```python
from build123d import *
from build123d.topology import SkipClean

# Parameters (mm, degrees)
SKETCH1_W           = 10
SKETCH1_H           = 10
BOSS_EXTRUDE1_DEPTH = 100
SKETCH2_W           = 25
SKETCH2_H           = 20
SKETCH2_R           = 1
BOSS_EXTRUDE2_DEPTH = 2
CUT_EXTRUDE2_DEPTH  = 2.5
CHAMFER2_SIZE       = 2.5
BOSS_EXTRUDE3_DEPTH = 7.5
CUT_EXTRUDE3_DEPTH  = 7.5
SKETCH8_W           = 40
SKETCH8_H           = 10
BOSS_EXTRUDE4_DEPTH = 3
FILLET1_R           = 2
SKETCH9_R           = 3
CUT_EXTRUDE4_DEPTH  = 5


with BuildPart() as part:
    # Sketch1 → Boss-Extrude1 (new, symmetric)
    with BuildSketch(Plane.XY):
        Rectangle(SKETCH1_W, SKETCH1_H)
    extrude(amount=BOSS_EXTRUDE1_DEPTH, both=True)

    # Sketch2 → Boss-Extrude2 (add)
    with BuildSketch(Plane(origin=(0, 0, -100), x_dir=(-1, 0, 0), z_dir=(0, 0, -1))):
        with Locations((0, 5)):
            Rectangle(SKETCH2_W, SKETCH2_H)
        with Locations((-8, 5.6)):
            Circle(SKETCH2_R, mode=Mode.SUBTRACT)
        with Locations(Location((8, 5.6, 0), (0, 0, 180))):
            Circle(SKETCH2_R, mode=Mode.SUBTRACT)
    extrude(amount=BOSS_EXTRUDE2_DEPTH)

    # Sketch4 → Cut-Extrude2 (cut)
    with BuildSketch(Plane(origin=(0, 5, 0), x_dir=(1, 0, 0), z_dir=(0, 1, 0))):
        Polygon((5, 100), (2.5, 100), (2.5, 92.5), (5, 90), (5, 92.5), align=None)
        Polygon((-5, 90), (-5, 92.5), (-5, 100), (-2.5, 100), (-2.5, 92.5), align=None)
    extrude(amount=-CUT_EXTRUDE2_DEPTH, mode=Mode.SUBTRACT)

    # Chamfer2
    chamfer2_edges = [part.edges().sort_by_distance(p)[0] for p in [
        (-2.5, 2.5, -96.25),
        (2.5, 2.5, -96.25),
    ]]
    chamfer(chamfer2_edges, length=CHAMFER2_SIZE - 0.0001)  # a hair under: the kernel refuses the full size

    # Sketch5 → Boss-Extrude3 (add)
    with SkipClean():  # the faces are left unmerged after this step: merging them gives an invalid solid
        with BuildSketch(Plane.XY.offset(-100)):
            Polygon((-2.5, 5), (-1, 6.5), (1, 6.5), (2.5, 5), align=None)
        extrude(amount=BOSS_EXTRUDE3_DEPTH)

    # Sketch7 → Cut-Extrude3 (cut)
    with SkipClean():  # the faces are left unmerged after this step: merging them gives an invalid solid
        with BuildSketch(Plane(origin=(5, 0, 0), x_dir=(0, 0, -1), z_dir=(1, 0, 0))):
            Polygon((92.5, 5), (94, 6.5), (92.5, 6.5), align=None)
        extrude(amount=-CUT_EXTRUDE3_DEPTH, mode=Mode.SUBTRACT)

    # Chamfer3: read off the stored shape, not the designer's step
    # Chamfer3: loft between two sections, ruled curve by curve
    with SkipClean():  # the faces are left unmerged after this step: merging them gives an invalid solid
        chamfer3_from = [
            Edge.make_line((-5, -5, -98.267949192), (-5, 2.5, -98.267949192)),
            Edge.make_line((-5, 2.5, -98.267949192), (-1, 6.5, -98.267949192)),
            Edge.make_line((-1, 6.5, -98.267949192), (1, 6.5, -98.267949192)),
            Edge.make_line((1, 6.5, -98.267949192), (5, 2.5, -98.267949192)),
            Edge.make_line((5, -5, -98.267949192), (5, 2.5, -98.267949192)),
            Edge.make_line((5, -5, -98.267949192), (-5, -5, -98.267949192)),
        ]
        chamfer3_to = [
            Edge.make_line((-6, -5, -100), (-6, 2.914213562, -100)),
            Edge.make_line((-6, 2.914213562, -100), (-1.414213562, 7.5, -100)),
            Edge.make_line((-1.414213562, 7.5, -100), (1.414213562, 7.5, -100)),
            Edge.make_line((1.414213562, 7.5, -100), (6, 2.914213562, -100)),
            Edge.make_line((6, -5, -100), (6, 2.914213562, -100)),
            Edge.make_line((6, -5, -100), (-6, -5, -100)),
        ]
        chamfer3 = Solid(Shell([*[Face.make_surface_from_curves(chamfer3_from[k], chamfer3_to[k]) for k in range(6)], Face(Wire(chamfer3_from)), Face(Wire(chamfer3_to))]))
        add(chamfer3)

    # Sketch8 → Boss-Extrude4 (add)
    with SkipClean():  # the faces are left unmerged after this step: merging them gives an invalid solid
        with BuildSketch(Plane(origin=(5, 0, 0), x_dir=(0, 0, -1), z_dir=(1, 0, 0))):
            Rectangle(SKETCH8_W, SKETCH8_H)
            with BuildLine():
                Line((0.419781931, 3.827046267), (16.278971963, 2.087479782))
                ThreePointArc((16.278971963, 2.087479782), (18.15, 0), (16.278971963, -2.087479782))
                Line((16.278971963, -2.087479782), (0.419781931, -3.827046267))
                ThreePointArc((0.419781931, -3.827046267), (0, -3.85), (-0.419781931, -3.827046267))
                Line((-0.419781931, -3.827046267), (-16.278971963, -2.087479782))
                ThreePointArc((-16.278971963, -2.087479782), (-18.15, 0), (-16.278971963, 2.087479782))
                Line((-16.278971963, 2.087479782), (-0.419781931, 3.827046267))
                ThreePointArc((-0.419781931, 3.827046267), (0, 3.85), (0.419781931, 3.827046267))
            make_face(mode=Mode.SUBTRACT)
        extrude(amount=BOSS_EXTRUDE4_DEPTH)

    # Fillet1
    # the kernel refuses this fillet: 2 mm, written as the material it takes off along each edge
    with BuildSketch(Plane(origin=(5, 5, -20), x_dir=(0, -1, 0), z_dir=(1, 0, 0)), Plane(origin=(5, -5, -20), x_dir=(0, 0, 1), z_dir=(1, 0, 0))) as fillet1_piece_1:
        with BuildLine():
            CenterArc((FILLET1_R, -FILLET1_R), FILLET1_R, 90, 90)
            Line((0, -FILLET1_R), (0, 0))
            Line((0, 0), (FILLET1_R, 0))
        make_face()
    extrude(amount=8, mode=Mode.SUBTRACT)
    with BuildSketch(Plane(origin=(5, 5, 20), x_dir=(0, -1, 0), z_dir=(1, 0, 0)), Plane(origin=(5, -5, 20), x_dir=(0, 0, -1), z_dir=(1, 0, 0))) as fillet1_piece_2:
        with BuildLine():
            CenterArc((FILLET1_R, FILLET1_R), FILLET1_R, 180, 90)
            Line((0, FILLET1_R), (0, 0))
            Line((0, 0), (FILLET1_R, 0))
        make_face()
    extrude(amount=8, mode=Mode.SUBTRACT)

    # Sketch9 → Cut-Extrude4 (cut)
    with SkipClean():  # the faces are left unmerged after this step: merging them gives an invalid solid
        with BuildSketch(Plane.ZY.offset(5)):
            Circle(SKETCH9_R)
        extrude(amount=-CUT_EXTRUDE4_DEPTH, mode=Mode.SUBTRACT)


solid = part.part
```
For this review, take the finished solid that the model builds, in its own axes (mm). A direction names the side the tool comes from. Round coordinates to 2 decimals unless told otherwise and drop trailing zeros. Write each loop counter-clockwise with the first axis right and the second up, starting at its lowest first coordinate (ties: lowest second). Pieces come first, ordered by that corner, then holes. Notation, with made-up numbers: (-24.5, 78.5) - (-16.5, 78.5) arc R14 cw to (-16.5, 89.5) - close; hole circle Ø4 at (5.25, 26.25). An arc over 180 degrees is marked (long way). Answer as CSV lines item,"result". Start each with the question number.
(1) Machinability: for faces 1 (the flat face through (0, 0, 0)), 2 (the flat face through (-5, 2.2, 2.3)), 3 (the flat face through (0, 5, 5)), 4 (the flat face through (8, 4.5, 0.3)), 5 (the flat face through (5, 0, 0)), which of the approach directions +Z, -Z, +X, -X, +Y, -Y give a long, thin tool a straight path to every point of the face, cutting with its end or side? Answer none if there is none.
(2) For pin 1 (3 mm diameter, centred on y = -0.5, z = 1.5, fed in from -X); pin 2 (1 mm diameter, centred on x = -8.5, y = 0, fed in from +Z); pin 3 (3.5 mm diameter, centred on x = 6.5, y = -1, fed in from +Z); pin 4 (10.5 mm diameter, centred on x = 1.5, z = 50.5, fed in from +Y), all flat-tipped, find the tip position at first contact; note any pin that passes through.
(3) Mouldability with a two-part tool opening along Y and no side actions: class faces 6 (the cylindrical face through (-3, 0, -3)), 7 (the flat face through (5, 0, 60)), 8 (the flat face through (1, -5, -1)) as +Y half, -Y half, draft (parallel to the pull), parting line (faces both ways), or undercut.
(4) Add section B-B, the plane y = 11.75. State the section outline as (x, z) points.
(5) Add section A-A, the plane z = 44. State the section outline as (x, y) points.
(6) For line 1 (Y direction, x = -8, z = -101); line 2 (Y direction, x = 7.5, z = -12.5); line 3 (X direction, y = 4.5, z = -27.5), list the stretches that pass through material, from the lowest coordinate up.
From the geometry:
1,face 1,"-X"
1,face 2,"+Z, -X, +Y, -Y"
1,face 3,"+Z, +X, -X, +Y"
1,face 4,"+Z, +X, +Y, -Y"
1,face 5,"+X"
2,pin 1,"stops at x = -5"
2,pin 2,"stops at z = -100"
2,pin 3,"stops at z = 100"
2,pin 4,"stops at y = 5"
3,face 6,"undercut"
3,face 7,"draft"
3,face 8,"-Y half"
4,outline,"(-12.5, -102) - (12.5, -102) - (12.5, -100) - (-12.5, -100) - close"
5,outline,"(-5, -5) - (5, -5) - (5, 5) - (-5, 5) - close"
6,line 1,"y = -5 to 4.6, 6.6 to 15"
6,line 2,"y = -5 to -2.5, 2.5 to 5"
6,line 3,"x = -5 to 5"
